Input: part model. Units: mm. Frame: model coordinates. Face numbers are marked on the shaded views. A direction names the side the tool comes from. Coordinates: 2 decimals unless noted, no trailing zeros. Order: outer loops, then holes, each group sorted by start corner. A loop starts at its lowest first (then second) coordinate and runs counter-clockwise, first axis right, second up. Notation, with made-up numbers: M 0,10.5 L 26,10.5 A16 ccw 26,20.5 Z; hole C -14,70 d3. An arc over 180 degrees is marked long. Answer in a Markdown table with one row per item.
from build123d import *

# Parameters (mm, degrees)
CROQUIS1_W              = 24
CROQUIS1_H              = 24
SALIENTE_EXTRUIR1_DEPTH = 15
CROQUIS2_W              = 20.3
CROQUIS2_H              = 20.3
CORTAR_EXTRUIR1_DEPTH   = 20
CORTAR_EXTRUIR2_REACH   = 32.741
CROQUIS3_R              = 2.25
CROQUIS4_W              = 5
CROQUIS4_H              = 15
SALIENTE_EXTRUIR2_DEPTH = 80
CROQUIS5_W              = 4
CROQUIS5_H              = 4
SALIENTE_EXTRUIR3_DEPTH = 15
REDONDEO1_START         = -1
REDONDEO1_DEPTH         = 17
REDONDEO1_2_DEPTH       = 15
CORTAR_EXTRUIR5_REACH   = 96.336
CROQUIS6_R              = 2.25
REDONDEO3_R             = 3


with BuildPart() as part:
    # Croquis1 → Saliente-Extruir1 (new body)
    with BuildSketch(Plane.XY):
        Rectangle(CROQUIS1_W, CROQUIS1_H)
    extrude(amount=SALIENTE_EXTRUIR1_DEPTH)

    # Croquis2 → Cortar-Extruir1 (cut)
    with BuildSketch(Plane(origin=(0, 0, 0), x_dir=(-1, 0, 0), z_dir=(0, 0, -1))):
        Rectangle(CROQUIS2_W, CROQUIS2_H)
    extrude(amount=-CORTAR_EXTRUIR1_DEPTH, mode=Mode.SUBTRACT)

    # Croquis3 → Cortar-Extruir2 (cut, up to next)
    with BuildSketch(Plane(origin=(0, 12, 0), x_dir=(1, 0, 0), z_dir=(0, 1, 0)), mode=Mode.PRIVATE) as cortar_extruir2_sk1:
        with Locations(Location((0, -7.5, 0), (0, 0, 270))):
            Circle(CROQUIS3_R)
    cortar_extruir2_tool1 = extrude(cortar_extruir2_sk1.sketch, amount=-CORTAR_EXTRUIR2_REACH, mode=Mode.PRIVATE) & part.part
    add(cortar_extruir2_tool1.solids().sort_by_distance((0, 12, 7.5))[0], mode=Mode.SUBTRACT)

    # Croquis4 → Saliente-Extruir2 (add)
    with BuildSketch(Plane.XZ.offset(12)):
        with Locations((0, 7.5)):
            Rectangle(CROQUIS4_W, CROQUIS4_H)
    extrude(amount=SALIENTE_EXTRUIR2_DEPTH)

    # Croquis5 → Saliente-Extruir3 (add)
    with BuildSketch(Plane.XY.offset(15)):
        with Locations((0, -8.15)):
            Rectangle(CROQUIS5_W, CROQUIS5_H)
    extrude(amount=-SALIENTE_EXTRUIR3_DEPTH)

    # Redondeo1: read off the stored shape, not the designer's step
    # Redondeo1 outline → Redondeo1 (cut)
    with BuildSketch(Plane.XY.offset(REDONDEO1_START)):
        with BuildLine():
            ThreePointArc((-2, -8.15), (-1.414213562, -6.735786438), (0, -6.15))
            Line((0, -6.15), (-2, -6.15))
            Line((-2, -6.15), (-2, -8.15))
        make_face()
        with BuildLine():
            ThreePointArc((0, -6.15), (1.414213562, -6.735786438), (2, -8.15))
            Line((2, -8.15), (2, -6.15))
            Line((2, -6.15), (0, -6.15))
        make_face()
    extrude(amount=REDONDEO1_DEPTH, mode=Mode.SUBTRACT)

    # Redondeo1 2 outline → Redondeo1 2 (add)
    with BuildSketch(Plane.XY):
        with BuildLine():
            Line((-2, -10.15), (-2, -8.15))
            ThreePointArc((-2, -8.15), (-2.585786438, -9.564213562), (-4, -10.15))
            Line((-4, -10.15), (-2, -10.15))
        make_face()
        with BuildLine():
            ThreePointArc((4, -10.15), (2.585786438, -9.564213562), (2, -8.15))
            Line((2, -8.15), (2, -10.15))
            Line((2, -10.15), (4, -10.15))
        make_face()
    extrude(amount=REDONDEO1_2_DEPTH)

    # Croquis6 → Cortar-Extruir5 (cut, up to next)
    with BuildSketch(Plane.ZY.offset(2.5), mode=Mode.PRIVATE) as cortar_extruir5_sk1:
        with Locations((7.5, -87)):
            Circle(CROQUIS6_R)
    cortar_extruir5_tool1 = extrude(cortar_extruir5_sk1.sketch, amount=-CORTAR_EXTRUIR5_REACH, mode=Mode.PRIVATE) & part.part
    add(cortar_extruir5_tool1.solids().sort_by_distance((-2.5, -87, 7.5))[0], mode=Mode.SUBTRACT)

    # Redondeo3
    redondeo3_edges = [part.edges().sort_by_distance(p)[0] for p in [
        (-2.5, -12, 7.5),
        (2.5, -12, 7.5),
    ]]
    fillet(redondeo3_edges, radius=REDONDEO3_R)


solid = part.part
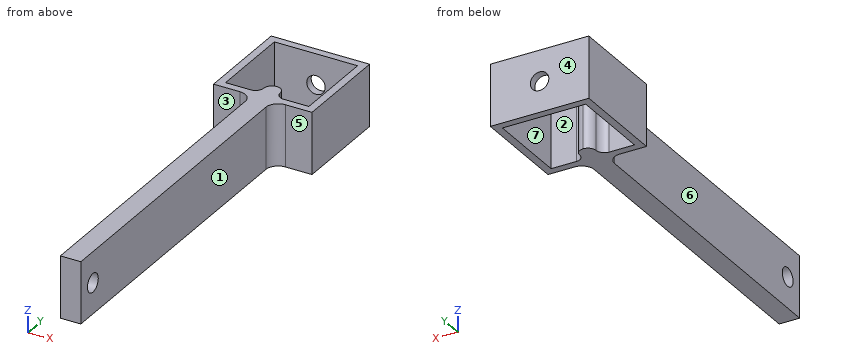
1) Cut plane C-C, the plane x = -8. Output: boundary loops of the cut face in (y, z).
Resolved:
| item | result |
|---|---|
| outline | M -12,0 L -10.15,0 L -10.15,15 L -12,15 Z; M 10.15,0 L 12,0 L 12,15 L 10.15,15 Z |
2) Cut plane B-B, the plane y = -87. Output: boundary loops of the cut face in (x, z), and give its area (3 significant figures).
Resolved:
| item | result |
|---|---|
| outline | M -2.5,0 L 2.5,0 L 2.5,5.25 L -2.5,5.25 Z; M -2.5,9.75 L 2.5,9.75 L 2.5,15 L -2.5,15 Z |
| area | 52.5 mm2 |
3) Reachability of the marked faces 1, 2 and 3 from +Z, -Z, +X, -X, +Y, -Y: full face, straight path, thin tool, end or side. Return the list, or none.
Resolved:
| item | result |
|---|---|
| face 1 | +Z, -Z, +X, -Y |
| face 2 | +Z, -Z |
| face 3 | +Z, -Z, -X, -Y |
4) Cut plane A-A, the plane z = 7.5. Output: boundary loops of the cut face in (x, y).
Resolved:
| item | result |
|---|---|
| outline | M -12,-12 L -5.5,-12 A3 cw -2.5,-15 L -2.5,-84.75 L 2.5,-84.75 L 2.5,-15 A3 cw 5.5,-12 L 12,-12 L 12,12 L 2.25,12 L 2.25,10.15 L 10.15,10.15 L 10.15,-10.15 L 4,-10.15 A2 cw 2,-8.15 A2 ccw -2,-8.15 A2 cw -4,-10.15 L -10.15,-10.15 L -10.15,10.15 L -2.25,10.15 L -2.25,12 L -12,12 Z; M -2.5,-92 L 2.5,-92 L 2.5,-89.25 L -2.5,-89.25 Z |
5) Mould query, pull axis Y, two halves, no side actions, for the marked faces 4, 5, 6 and 7. Classes: +Y half, -Y half, draft (parallel to the pull), parting line (faces both ways), or undercut.
Resolved:
| item | result |
|---|---|
| face 4 | +Y half |
| face 5 | -Y half |
| face 6 | draft |
| face 7 | undercut |
6) Material intervals for probe 1 along Y at (x, z) = (-7.75, 1.75); probe 2 along X at (y, z) = (-24, 1.75), sorted ascending.
Resolved:
| item | result |
|---|---|
| probe 1 | y = -12 to -10.15, 10.15 to 12 |
| probe 2 | x = -2.5 to 2.5 |
7) Cut plane D-D, the plane y = -54. Output: boundary loops of the cut face in (x, z).
Resolved:
| item | result |
|---|---|
| outline | M -2.5,0 L 2.5,0 L 2.5,15 L -2.5,15 Z |
8) Contact query for flat-ended pins moving along their axis: pin 1 (2 mm diameter, centred on x = -8, z = 11, fed in from -Y); pin 2 (7.5 mm diameter, centred on y = -38, z = 4.5, fed in from -X); pin 3 (2 mm diameter, centred on y = -48.5, z = 11.5, fed in from +X). Output: stop coordinate, or through.
Resolved:
| item | result |
|---|---|
| pin 1 | stops at y = -12 |
| pin 2 | stops at x = -2.5 |
| pin 3 | stops at x = 2.5 |
